Can you work these out from the model? Positions are in its coordinate system, mm. Face numbers are marked on the shaded views. A direction names the side the tool comes from. Round coordinates to 2 decimals unless told otherwise and drop trailing zeros. Loops run counter-clockwise (first coordinate to the right, second up) from the corner with the lowest first, then second, coordinate; pieces in that order, holes last.
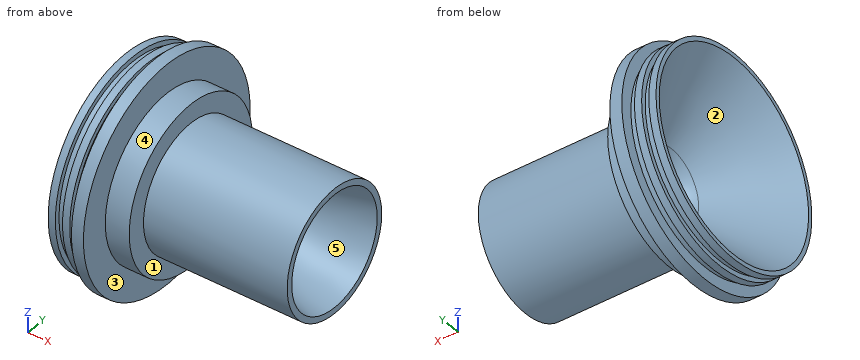
from build123d import *


with BuildPart() as part:
    # Sketch1 → Revolve1 (revolve)
    with BuildSketch(Plane.XY):
        with BuildLine():
            Line((-87, 41.080611397), (-60.892786886, 14.973398282))
            ThreePointArc((-60.892786886, 14.973398282), (-54.168470844, 11.091112606), (-46.403899491, 11.091112606))
            Line((-46.403899491, 11.091112606), (0, 23.525))
            Line((0, 23.525), (0, 26))
            Line((0, 26), (-60, 26))
            Line((-60, 26), (-60, 33.85))
            Line((-60, 33.85), (-70, 33.85))
            Line((-70, 33.85), (-70, 45.85))
            Line((-70, 45.85), (-75, 45.85))
            Line((-75, 45.85), (-75, 40.86))
            Line((-75, 40.86), (-78, 40.86))
            Line((-78, 40.86), (-78, 42.86))
            Line((-78, 42.86), (-81, 42.86))
            Line((-81, 42.86), (-81, 40.86))
            Line((-81, 40.86), (-84, 40.86))
            Line((-84, 40.86), (-84, 42.86))
            Line((-84, 42.86), (-87, 42.86))
            Line((-87, 42.86), (-87, 41.080611397))
        make_face()
    revolve(axis=Axis((0, 0, 0), (-1, 0, 0)))


solid = part.part
(1) If we section it at A-A, the plane x = -30: List the corners of the cut face in (y, z) for me.
Worked answers:
outline: circle Ø52 at (0, 0); hole circle Ø30.97 at (0, 0)
(2) If we mould it in two halves opening along Y, with no side actions, what happens to the marked faces 3, 4 and 5? For each: released by +Y, released by -Y, zero draft, split by the parting line, or undercut.
Worked answers:
face 3: zero draft
face 4: split by the parting line
face 5: undercut
(3) Will these pins go through, and if not, where does the flat tip stop? P1, Ø6, axis at x = -36, y = 3, coming from the +Z side; P2, Ø8, axis at x = -54.5, z = 32, coming from the -Y side; P3, Ø5, axis at x = -10.5, y = -13.5, coming from the -Z side; P4, Ø8, axis at x = -60.5, z = 31.5, coming from the +Y side.
Worked answers:
P1: stops at z = 26
P2: passes through
P3: stops at z = -23.56
P4: stops at y = 19.74
(4) If we section it at B-B, the plane x = -12: List the corners of the cut face in (y, z) for me, then the cut area to 3 significant figures.
Worked answers:
outline: circle Ø52 at (0, 0); hole circle Ø40.62 at (0, 0)
area: 828 mm2
(5) If I drill on line 1 (X direction, y = -13, z = 40); line 2 (Y direction, x = -70.5, z = -18); line 3 (X direction, y = -25, z = -37), over which ranges is the centre line in solid material (lowest first)?
Worked answers:
line 1: x = -87 to -84, -81 to -78, -75 to -70
line 2: y = -42.17 to -16.74, 16.74 to 42.17
line 3: x = -75 to -70
(6) For the marked faces 1 and 2, which set-ups out of +Z, -Z, +X, -X, +Y, -Y let a thin tool reach every point of the face, with its end or its side?
Worked answers:
face 1: +X
face 2: -X
